Drawing for the job (mm, zero at the part's lowest x, y, z). Give positions to 0.01 mm unless a question says otherwise; leave off trailing zeros. Write each loop counter-clockwise with the first axis right and the second up, starting at its lowest first coordinate (ties: lowest second). Pieces come first, ordered by that corner, then holes.
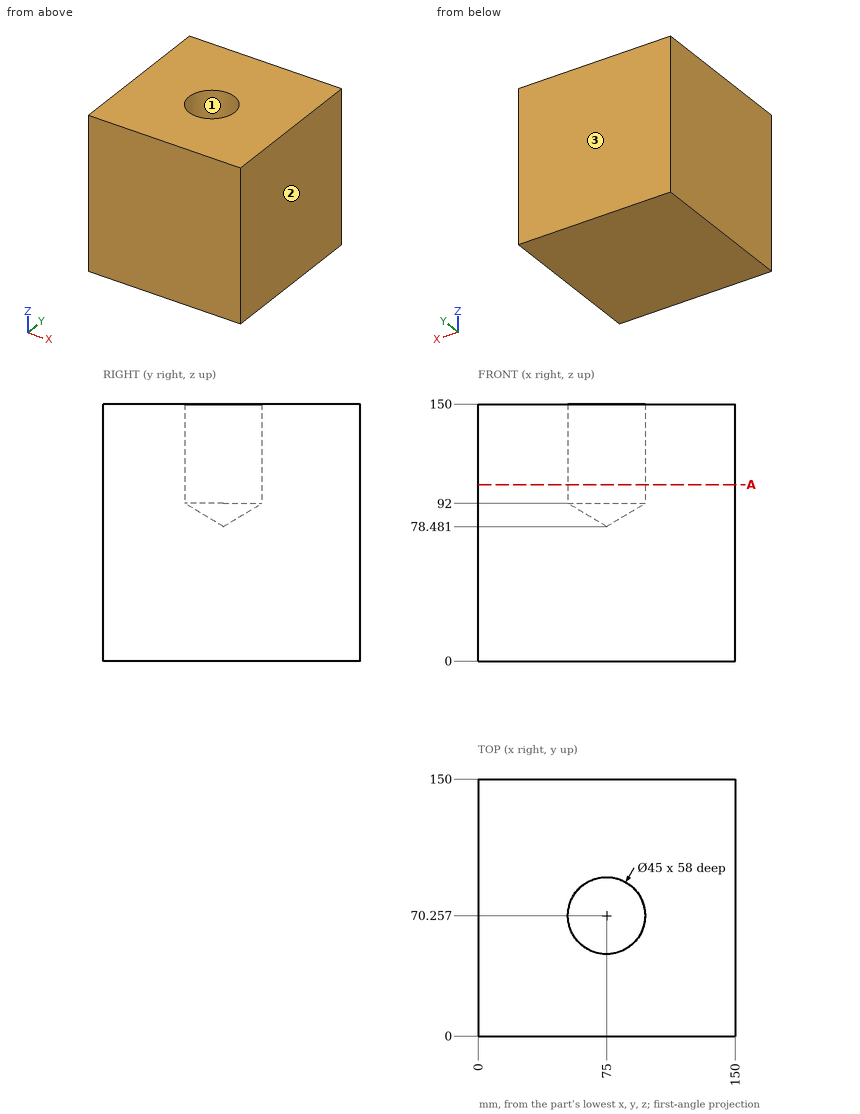
1. Pin check, flat tip, straight feed: P1, Ø1, axis at x = 73.5, y = 55, coming from the +Z side. Stop position of the tip, or through.
Calculated:
P1: stops at z = 87.99
2. Probe probe 1 along Y at (x, z) = (75, 113); probe 2 along Y at (x, z) = (76, 82) (1 decimal); probe 3 along X at (y, z) = (77.5, 111.5). List the from-to ranges inside material, lowest first.
Calculated:
probe 1: y = 0 to 47.76, 92.76 to 150
probe 2: y = 0 to 64.5, 76 to 150
probe 3: x = 0 to 53.7, 96.3 to 150
3. Slice it at A-A, the plane z = 103. Write the cut outline in (x, y).
Calculated:
outline: (0, 0) - (150, 0) - (150, 150) - (0, 150) - close; hole circle Ø45 at (75, 70.26)
4. Pull direction Y, two halves, no side cores. Call the marked faces 1, 2 and 3: +Y half, -Y half, draft (parallel to the pull), parting line (faces both ways), or undercut.
Calculated:
face 1: undercut
face 2: draft
face 3: +Y half
